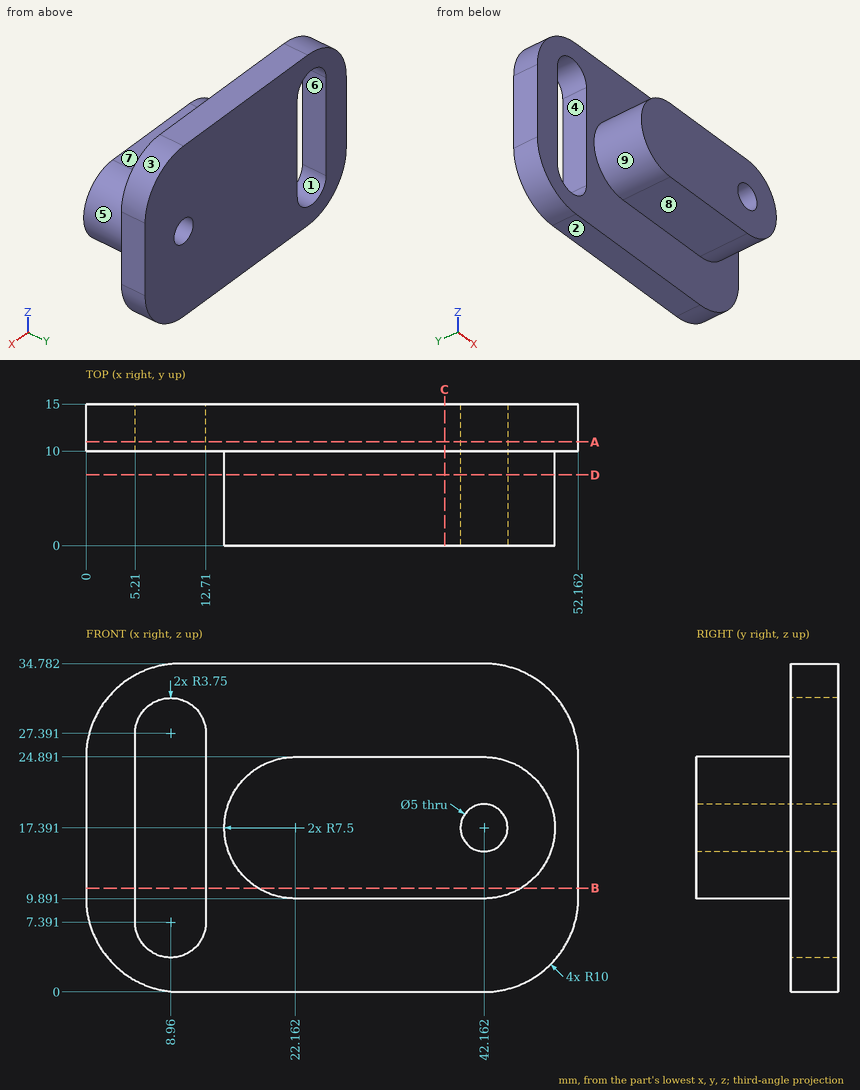
Print and shaded views of the part. All mm, measured from the part's lowest x, y and z. A direction names the side the tool comes from. Round coordinates to 2 decimals unless told otherwise and drop trailing zeros. Write each loop counter-clockwise with the first axis right and the second up, starting at its lowest first coordinate (ties: lowest second). Pieces come first, ordered by that corner, then holes. Notation, with made-up numbers: (39, 20) - (49, 20) arc R17 cw to (49, 38) - close; hole circle Ø1 at (68, -23.5). An arc over 180 degrees is marked (long way). One line per item, written item: value.
(1) Cut at A-A, the plane y = 11. Give the cut face in (x, z), plus the area to 3 significant figures.
Values follow:
outline: (0, 10) arc R10 ccw to (10, 0) - (42.16, 0) arc R10 ccw to (52.16, 10) - (52.16, 24.78) arc R10 ccw to (42.16, 34.78) - (10, 34.78) arc R10 ccw to (0, 24.78) - close; hole (5.21, 7.39) arc R3.75 ccw to (12.71, 7.39) - (12.71, 27.39) arc R3.75 ccw to (5.21, 27.39) - close; hole circle Ø5 at (42.16, 17.39)
area: 1,510 mm²
(2) Wall check: probe 1 along Z at (x, y) = (32.5, 3.5); probe 2 along Y at (x, z) = (26, 26); probe 3 along Z at (x, y) = (8.5, 13.25). Give the ranges that are in metal, low to high.
Values follow:
probe 1: z = 9.89 to 24.89
probe 2: y = 10 to 15
probe 3: z = 0.11 to 3.67, 31.11 to 34.67
(3) Cut at B-B, the plane z = 11. Give the cut face in (x, y), plus the area to 3 significant figures.
Values follow:
outline: (0, 10) - (5.21, 10) - (5.21, 15) - (0, 15) - close; (12.71, 10) - (18.24, 10) - (18.24, 0) - (46.09, 0) - (46.09, 10) - (52.16, 10) - (52.16, 15) - (12.71, 15) - close
area: 502 mm²
(4) Cut at C-C, the plane x = 38. Give the cut face in (y, z), plus the area to 3 significant figures.
Values follow:
outline: (0, 9.89) - (10, 9.89) - (10, 0) - (15, 0) - (15, 34.78) - (10, 34.78) - (10, 24.89) - (0, 24.89) - close
area: 324 mm²
(5) Two-plate mould, pull along Z, no slides. Class the marked faces 1, 2, 3 and 4: pulls with the +Z half, pulls with the -Z half, needs draft (parallel to the pull), parting line crosses it, or undercut.
Values follow:
face 1: undercut
face 2: pulls with the -Z half
face 3: pulls with the +Z half
face 4: undercut
(6) 3-axis set-ups, long thin cutter, end or side, ignore diameter. For the marked faces 5, 6, 7, 8 and 9: which of +Z, -Z, +X, -X, +Y, -Y reach the whole face in a straight line?
Values follow:
face 5: +X, -Y
face 6: +Y, -Y
face 7: +Z, +X, -X, -Y
face 8: -Z, +X, -X, -Y
face 9: -X, -Y
(7) Drop flat-ended pins along their axis: P1, Ø6, axis at y = 2.5, z = 15, coming from the -X side; P2, Ø1, axis at x = 19, z = 5, coming from the -Y side; P3, Ø3, axis at y = 5.5, z = 9, coming from the -X side. Give the stop position or say it passes through.
Values follow:
P1: stops at x = 14.66
P2: stops at y = 10
P3: stops at x = 19.2
(8) Cut at D-D, the plane y = 7.5. Give the cut face in (x, z), plus the area to 3 significant figures.
Values follow:
outline: (22.16, 9.89) - (42.16, 9.89) arc R7.5 ccw to (42.16, 24.89) - (22.16, 24.89) arc R7.5 ccw to start; hole circle Ø5 at (42.16, 17.39)
area: 457 mm²
